Source: CAD feature listing. Evaluate the final solid. Frame: model axes, mm. A direction names the side the tool comes from. Round coordinates to 2 decimals unless told otherwise and drop trailing zeros. Loops run counter-clockwise (first coordinate to the right, second up) from the corner with the lowest first, then second, coordinate; pieces in that order, holes last.
Item 1: Section query A-A on x = -5.75. Return loops of the section in (y, z), then the cut area to 3 significant figures.
Item 2: First-contact query: P1, Ø0.8, axis at x = 0.5, z = 199, coming from the -Y side; P2, Ø4, axis at y = 92.5, z = 129.5, coming from the -X side; P3, Ø0.5, axis at x = 1, z = 199, coming from the +Y side. Flat tips, straight axial feed; report the tip coordinate or a pass-through.
Item 3: Ray query, L1, parallel to Y at x = -7.75, z = 84.5; L2, parallel to Z at x = -2.75, y = 176; L3, parallel to X at y = 23.5, z = 46.5. Return the intervals inside material, ascending.
Item 4: Access query for faces 5 (the flat face through (1.5, 104, 97)), 6 (the flat face through (-5, 1.5, 99)), 7 (the flat face through (-10, 104, 198.5)). Directions: +Z, -Z, +X, -X, +Y, -Y. A direction counts if a zero-diameter tool reaches every point of the face in a straight line with its end or side. Return the directions, or none.
Item 5: Section query B-B on y = 125.5. Return loops of the section in (x, z), then the cut area to 3 significant figures.
Item 6: Pull-direction query (Y, two-part tool) for faces 1 (the flat face through (-5, 208.5, 101)), 2 (the flat face through (-5, 210, 101)), 3 (the flat face through (0, 104, 97)), 4 (the flat face through (-5, 0, 99)); classes: released by +Y, released by -Y, zero draft, split by the parting line, or undercut.
Item 7: Section query C-C on z = 106. Return loops of the section in (x, y), then the cut area to 3 significant figures.
```python
from build123d import *

# Parameters (mm, degrees)
SKETCH_2_W                       = 1.5
SKETCH_2_H                       = 210
SM_BASE_FLANGE_1_DEPTH           = 200
SM_EDGE_FLANGE_1_STRIP_W         = 7.4732
SM_EDGE_FLANGE_1_STRIP_H         = 1.5
SM_EDGE_FLANGE_1_STRIP_CUT_DEPTH = 200
SM_EDGE_FLANGE_1_DEPTH           = 200
SM_EDGE_FLANGE_2_STRIP_W         = 7.4732
SM_EDGE_FLANGE_2_STRIP_H         = 1.5
SM_EDGE_FLANGE_2_STRIP_CUT_DEPTH = 200
SM_EDGE_FLANGE_2_DEPTH           = 200
SM_EDGE_FLANGE_3_STRIP_W         = 7.4732
SM_EDGE_FLANGE_3_STRIP_H         = 1.5
SM_EDGE_FLANGE_3_STRIP_CUT_DEPTH = 205.5268
SM_EDGE_FLANGE_3_DEPTH           = 205.5268


# Sheet-metal steps are written as plain solids
with BuildPart() as part:
    # Sketch 2 → 基体-法兰1 (new body)
    with BuildSketch(Plane.XY):
        with Locations((0.75, 105)):
            Rectangle(SKETCH_2_W, SKETCH_2_H)
    extrude(amount=SM_BASE_FLANGE_1_DEPTH)

    # 边线-法兰1 strip (across the edge) → 边线-法兰1 strip cut (cut)
    with BuildSketch(Plane(origin=(0, 210, 200), x_dir=(0, -1, 0), z_dir=(0, 0, -1))):
        with Locations((-1.5, -0.75)):
            Rectangle(SM_EDGE_FLANGE_1_STRIP_W, SM_EDGE_FLANGE_1_STRIP_H)
    extrude(amount=SM_EDGE_FLANGE_1_STRIP_CUT_DEPTH, mode=Mode.SUBTRACT)

    # 边线-法兰1 section (across the edge) → 边线-法兰1 (add)
    with BuildSketch(Plane(origin=(0, 210, 200), x_dir=(0, -1, 0), z_dir=(0, 0, -1))):
        with BuildLine():
            Line((0, 0.7366), (0, 8.5))
            Line((0, 8.5), (1.5, 8.5))
            Line((1.5, 8.5), (1.5, 0.7366))
            ThreePointArc((1.5, 0.7366), (1.715745145, 0.215745145), (2.2366, 0))
            Line((2.2366, 0), (2.2366, -1.5))
            ThreePointArc((2.2366, -1.5), (0.655084973, -0.844915027), (0, 0.7366))
        make_face()
    extrude(amount=SM_EDGE_FLANGE_1_DEPTH)

    # 边线-法兰2 strip (across the edge) → 边线-法兰2 strip cut (cut)
    with BuildSketch(Plane(origin=(0, 0, 0), x_dir=(0, 1, 0), z_dir=(0, 0, 1))):
        with Locations((-1.5, -0.75)):
            Rectangle(SM_EDGE_FLANGE_2_STRIP_W, SM_EDGE_FLANGE_2_STRIP_H)
    extrude(amount=SM_EDGE_FLANGE_2_STRIP_CUT_DEPTH, mode=Mode.SUBTRACT)

    # 边线-法兰2 section (across the edge) → 边线-法兰2 (add)
    with BuildSketch(Plane(origin=(0, 0, 0), x_dir=(0, 1, 0), z_dir=(0, 0, 1))):
        with BuildLine():
            Line((0, 0.7366), (0, 8.5))
            Line((0, 8.5), (1.5, 8.5))
            Line((1.5, 8.5), (1.5, 0.7366))
            ThreePointArc((1.5, 0.7366), (1.715745145, 0.215745145), (2.2366, 0))
            Line((2.2366, 0), (2.2366, -1.5))
            ThreePointArc((2.2366, -1.5), (0.655084973, -0.844915027), (0, 0.7366))
        make_face()
    extrude(amount=SM_EDGE_FLANGE_2_DEPTH)

    # 边线-法兰3 strip (across the edge) → 边线-法兰3 strip cut (cut)
    with BuildSketch(Plane(origin=(0, 2.2366, 200), x_dir=(0, 0, -1), z_dir=(0, 1, 0))):
        with Locations((-1.5, -0.75)):
            Rectangle(SM_EDGE_FLANGE_3_STRIP_W, SM_EDGE_FLANGE_3_STRIP_H)
    extrude(amount=SM_EDGE_FLANGE_3_STRIP_CUT_DEPTH, mode=Mode.SUBTRACT)

    # 边线-法兰3 section (across the edge) → 边线-法兰3 (add)
    with BuildSketch(Plane(origin=(0, 2.2366, 200), x_dir=(0, 0, -1), z_dir=(0, 1, 0))):
        with BuildLine():
            Line((0, 0.7366), (0, 18.5))
            Line((0, 18.5), (1.5, 18.5))
            Line((1.5, 18.5), (1.5, 0.7366))
            ThreePointArc((1.5, 0.7366), (1.715745145, 0.215745145), (2.2366, 0))
            Line((2.2366, 0), (2.2366, -1.5))
            ThreePointArc((2.2366, -1.5), (0.655084973, -0.844915027), (0, 0.7366))
        make_face()
    extrude(amount=SM_EDGE_FLANGE_3_DEPTH)


solid = part.part
```
Data:
1. outline: (0, 0) - (1.5, 0) - (1.5, 200) - (0, 200) - close; (2.24, 198.5) - (207.76, 198.5) - (207.76, 200) - (2.24, 200) - close; (208.5, 0) - (210, 0) - (210, 200) - (208.5, 200) - close
1. area: 908 mm2
2. P1: stops at y = 0.16
2. P2: stops at x = 0
2. P3: stops at y = 209.43
3. L1: y = 0 to 1.5, 208.5 to 210
3. L2: z = 198.5 to 200
3. L3: x = 0 to 1.5
4. face 5: +Z, -Z, +X, +Y, -Y
4. face 6: +Z, -Z, -X
4. face 7: -Z, -X
5. outline: (-18.5, 198.5) - (-0.74, 198.5) arc R0.74 cw to (0, 197.76) - (0, 0) - (1.5, 0) - (1.5, 197.76) arc R2.24 ccw to (-0.74, 200) - (-18.5, 200) - close
5. area: 327 mm2
6. face 1: undercut
6. face 2: released by +Y
6. face 3: undercut
6. face 4: released by -Y
7. outline: (-8.5, 0) - (-0.74, 0) arc R2.24 ccw to (1.5, 2.24) - (1.5, 207.76) arc R2.24 ccw to (-0.74, 210) - (-8.5, 210) - (-8.5, 208.5) - (-0.74, 208.5) arc R0.74 cw to (0, 207.76) - (0, 2.24) arc R0.74 cw to (-0.74, 1.5) - (-8.5, 1.5) - close
7. area: 339 mm2
